The model under review builds one solid part; all positions refer to its coordinate system, in mm. Face numbers are marked on the shaded views. A direction names the side the tool comes from. Coordinates: 2 decimals unless noted, no trailing zeros. Order: outer loops, then holes, each group sorted by start corner. A loop starts at its lowest first (then second) coordinate and runs counter-clockwise, first axis right, second up. Notation, with made-up numbers: (62.25, 69) - (110.25, 69) arc R26 cw to (110.25, 107) - close; hole circle Ø8 at (49.5, 21). An arc over 180 degrees is marked (long way). Answer in a Markdown table with one row per item.
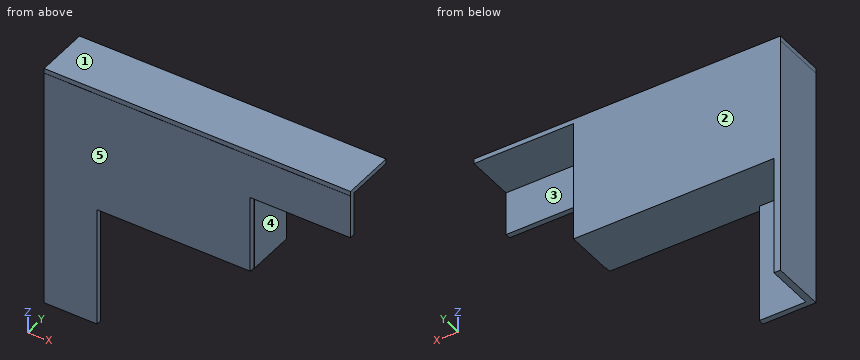
```python
from build123d import *

# Parameters (mm, degrees)
F0_W     = 116.2599772215
F0_H     = 70.1507925987
F1_DEPTH = 27.94
F2_W     = 3.7873648107
F2_H     = 27.94
F3_DEPTH = 139.7
F4_W     = 28.065841645
F4_H     = 2.7693584561
F4_W_2   = 3.0061341822
F5_DEPTH = 177.8
F7_DEPTH = 88.9


with BuildPart() as f1:
    # F0 (on Front) → F1 (new body)
    with BuildSketch(Plane.XZ):
        Rectangle(F0_W, F0_H)
    extrude(amount=F1_DEPTH)

    # F2 (on face) → F3 (join)
    with BuildSketch(Plane.XY.offset(35.0753962994)):
        with Locations((-60.0236710161, -13.97)):
            Rectangle(F2_W, F2_H)
        Polygon((-31.1518013477, -27.94), (-58.1299886107, -27.94), (-61.9173534214, -27.94), (-61.9173534214, -31.1609115452), (-31.1518013477, -31.1609115452), align=None)
    extrude(amount=-F3_DEPTH)

    # F4 (on face) → F5 (join)
    with BuildSketch(Plane(origin=(-61.9173534214, 0, 0), x_dir=(0, -1, 0), z_dir=(-1, 0, 0))):
        with Locations((14.0329208225, 36.4600755274)):
            Rectangle(F4_W, F4_H)
        Polygon((31.0719758272, 35.0753962994), (28.065841645, 35.0753962994), (28.065841645, 9.7159240395), (31.1609115452, 9.7159240395), (31.1609115452, 35.0753962994), align=None)
        with Locations((29.5689087361, 36.4600755274)):
            Rectangle(F4_W_2, F4_H)
    extrude(amount=-F5_DEPTH)

    # F6 (on face) → F7 (join)
    with BuildSketch(Plane.YZ.offset(-31.1518013477)):
        Polygon((-28.065841645, 9.7159240395), (-31.1609115452, 9.7159240395), (-31.1609115452, -35.0753962994), (-27.94, -35.0753962994), (-27.94, 9.7159240395), align=None)
    extrude(amount=F7_DEPTH)


solid = f1.part
```
Item 1: To check wall thickness, follow line 1 (Z direction, x = -31, y = -6); line 2 (Z direction, x = 78, y = -1.5); line 3 (X direction, y = -29, z = 7.5). State the ranges of each line that lie inside material, in increasing order. Write a range as from..to.
Check values:
| item | result |
|---|---|
| line 1 | -35.08..37.84 |
| line 2 | 35.08..37.84 |
| line 3 | -61.92..57.75 |
Item 2: Tool access review of the marked faces 4 and 5: name each direction out of +Z, -Z, +X, -X, +Y, -Y from which nothing blocks a thin tool from reaching the whole face with its end or side.
Check values:
| item | result |
|---|---|
| face 4 | -Z, +X, +Y |
| face 5 | +Z, -Z, +X, -X, -Y |
Item 3: We need section D-D, the plane x = 64. Write out the cut boundary in (y, z), then the cut area to 3 significant figures.
Check values:
| item | result |
|---|---|
| outline | (-31.16, 9.72) - (-28.07, 9.72) - (-28.07, 35.08) - (0, 35.08) - (0, 37.84) - (-31.07, 37.84) - (-31.07, 35.08) - (-31.16, 35.08) - close |
| area | 165 mm^2 |
Item 4: Clearance check with flat-ended pins moving along their axes: pin 1 Ø2.5 at (y, z) = (-30, -8) entering from +X; pin 2 Ø8.5 at (y, z) = (-16.5, 3.5) entering from +X; pin 3 Ø8.5 at (y, z) = (-13, -70) entering from +X. State where each tip first meets the part, or that it passes through.
Check values:
| item | result |
|---|---|
| pin 1 | x = 57.75 |
| pin 2 | x = 58.13 |
| pin 3 | x = -58.13 |
Item 5: We need section B-B, the plane z = -76. Write out the cut boundary in (x, y), then the cut area to 3 significant figures.
Check values:
| item | result |
|---|---|
| outline | (-61.92, -31.16) - (-31.15, -31.16) - (-31.15, -27.94) - (-58.13, -27.94) - (-58.13, 0) - (-61.92, 0) - close |
| area | 205 mm^2 |
Item 6: We need section C-C, the plane y = -21. Write out the cut boundary in (x, z).
Check values:
| item | result |
|---|---|
| outline | (-61.92, -104.62) - (-58.13, -104.62) - (-58.13, -35.08) - (58.13, -35.08) - (58.13, 35.08) - (115.88, 35.08) - (115.88, 37.84) - (-61.92, 37.84) - close |
Item 7: We need section A-A, the plane x = 30. Write out the cut boundary in (y, z).
Check values:
| item | result |
|---|---|
| outline | (-31.16, -35.08) - (0, -35.08) - (0, 37.84) - (-31.07, 37.84) - (-31.07, 35.08) - (-31.16, 35.08) - close; hole (-28.07, 9.72) - (-27.94, 9.72) - (-27.94, 35.08) - (-28.07, 35.08) - close |
Item 8: Mouldability with a two-part tool opening along Z and no side actions: class the marked faces 1, 2 and 3 as +Z half, -Z half, draft (parallel to the pull), parting line (faces both ways), or undercut.
Check values:
| item | result |
|---|---|
| face 1 | +Z half |
| face 2 | draft |
| face 3 | undercut |
